```python
from build123d import *

# Parameters (mm, degrees)
F0_W      = 13.2
F0_H      = 18.5
F1_DEPTH  = 26.5
F2_W      = 4
F2_H      = 4.5
F2_W_2    = 1.5
F3_DEPTH  = 18.501
F4_W      = 5
F4_H      = 2.5
F5_DEPTH  = 1.5
F6_W      = 6.5
F6_H      = 4
F7_DEPTH  = 13.201
F8_W      = 3.5
F8_H      = 8
F9_DEPTH  = 18.5
F10_R     = 2.5
F11_DEPTH = 26.501
F12_W     = 5.5
F12_H     = 4.75
F13_DEPTH = 26.501


with BuildPart() as f1:
    # F0 (on Front) → F1 (new body)
    with BuildSketch(Plane.XZ):
        Rectangle(F0_W, F0_H)
    extrude(amount=F1_DEPTH)

    # F2 (on face) → F3 (cut, through all)
    with BuildSketch(Plane.XY.offset(9.25)):
        with Locations((4.6, -2.25)):
            Rectangle(F2_W, F2_H)
        with Locations((-5.85, -2.25)):
            Rectangle(F2_W_2, F2_H)
    extrude(amount=-F3_DEPTH, mode=Mode.SUBTRACT)

    # F4 (on face) → F5 (join)
    with BuildSketch(Plane.YZ.offset(6.6)):
        with Locations((-12.5, 0)):
            Rectangle(F4_W, F4_H)
    extrude(amount=F5_DEPTH)

    # F6 (on face) → F7 (cut, through all)
    with BuildSketch(Plane.YZ.offset(6.6)):
        Polygon((-4.5, -9.25), (0, -9.25), (0, -5.75), (-6.5, -5.75), (-6.5, -9.25), align=None)
        with Locations((-3.25, 7.25)):
            Rectangle(F6_W, F6_H)
    extrude(amount=-F7_DEPTH, mode=Mode.SUBTRACT)

    # F8 (on face) → F9 (join, through all)
    with BuildSketch(Plane.XY.offset(9.25)):
        with Locations((8.35, -22.5)):
            Rectangle(F8_W, F8_H)
    extrude(amount=-F9_DEPTH)

    # F10 (on face) → F11 (cut, through all)
    with BuildSketch(Plane.XZ.offset(26.5)):
        with Locations((-0.6, 0.75)):
            Circle(F10_R)
    extrude(amount=-F11_DEPTH, mode=Mode.SUBTRACT)

    # F12 (on face) → F13 (cut, through all)
    with BuildSketch(Plane.XZ.offset(26.5)):
        with Locations((7.35, 6.875)):
            Rectangle(F12_W, F12_H)
        with Locations((7.35, -6.875)):
            Rectangle(F12_W, F12_H)
    extrude(amount=-F13_DEPTH, mode=Mode.SUBTRACT)


solid = f1.part
```
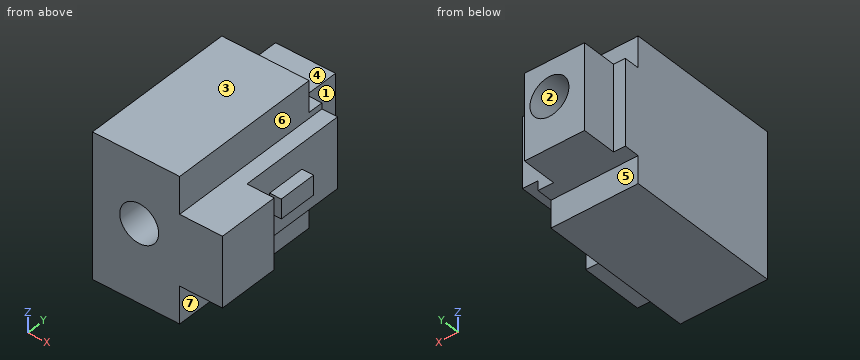
CAD build for the part. Positions are in the model's coordinates, mm. Face numbers are marked on the shaded views. A direction names the side the tool comes from. Round coordinates to 2 decimals unless told otherwise and drop trailing zeros. Order: outer loops, then holes, each group sorted by start corner. A loop starts at its lowest first (then second) coordinate and runs counter-clockwise, first axis right, second up.
Item 1: Saw through at B-B on x = -0.6. Write the cut outline in (y, z).
Item 2: Saw through at C-C on y = -12.5. Write the cut outline in (x, z).
Item 3: Tool access for the marked faces 4, 5, 6 and 7: list every direction of +Z, -Z, +X, -X, +Y, -Y with a clear straight run to the whole face (end or side of a thin tool).
Item 4: Probe line 1 along Z through (x, y) = (-0.6, -14.75); line 2 along Y through (x, z) = (-6, 4); line 3 along Y through (x, z) = (3, 5.75). List the from-to ranges inside material, lowest first.
Item 5: Saw through at A-A on z = 0.75. Write the cut outline in (x, y).
Item 6: Pin check, flat tips, straight feed: pin 1 (2 mm diameter, centred on x = -1.5, z = 6.5, fed in from +Y); pin 2 (3 mm diameter, centred on x = 7, z = 2, fed in from +Y); pin 3 (4.5 mm diameter, centred on x = 8, y = -14.5, fed in from -Z). Stop position of each tip, or through.
Item 7: Mould opens along Z. For the marked faces 1, 2 and 3 say: pulls with the +Z half, pulls with the -Z half, needs draft (parallel to the pull), parting line crosses it, or undercut.
Item 8: Saw through at D-D on x = -4.75. Write the cut outline in (y, z), then the cut area to 4 significant figures.
Reported:
1. outline: (-26.5, -9.25) - (-6.5, -9.25) - (-6.5, -5.75) - (0, -5.75) - (0, -1.75) - (-26.5, -1.75) - close; (-26.5, 3.25) - (0, 3.25) - (0, 5.25) - (-6.5, 5.25) - (-6.5, 9.25) - (-26.5, 9.25) - close
2. outline: (-6.6, -9.25) - (4.6, -9.25) - (4.6, -4.5) - (6.6, -4.5) - (6.6, -1.25) - (8.1, -1.25) - (8.1, 1.25) - (6.6, 1.25) - (6.6, 4.5) - (4.6, 4.5) - (4.6, 9.25) - (-6.6, 9.25) - close; hole circle Ø5 at (-0.6, 0.75)
3. face 4: +Z, +X, -X, +Y
3. face 5: -Z, +X, -X, +Y
3. face 6: +Z, +X, +Y, -Y
3. face 7: -Z, +X, +Y, -Y
4. line 1: z = -9.25 to -1.75, 3.25 to 9.25
4. line 2: y = -26.5 to -4.5
4. line 3: y = -26.5 to -6.5
5. outline: (-6.6, -26.5) - (-3.1, -26.5) - (-3.1, 0) - (-5.1, 0) - (-5.1, -4.5) - (-6.6, -4.5) - close; (1.9, -26.5) - (10.1, -26.5) - (10.1, -18.5) - (6.6, -18.5) - (6.6, -15) - (8.1, -15) - (8.1, -10) - (6.6, -10) - (6.6, -4.5) - (2.6, -4.5) - (2.6, 0) - (1.9, 0) - close
6. pin 1: stops at y = -6.5
6. pin 2: stops at y = -4.5
6. pin 3: stops at z = -4.5
7. face 1: needs draft
7. face 2: undercut
7. face 3: pulls with the +Z half
8. outline: (-26.5, -9.25) - (-6.5, -9.25) - (-6.5, -5.75) - (0, -5.75) - (0, 5.25) - (-6.5, 5.25) - (-6.5, 9.25) - (-26.5, 9.25) - close
8. area: 441.5 mm2
